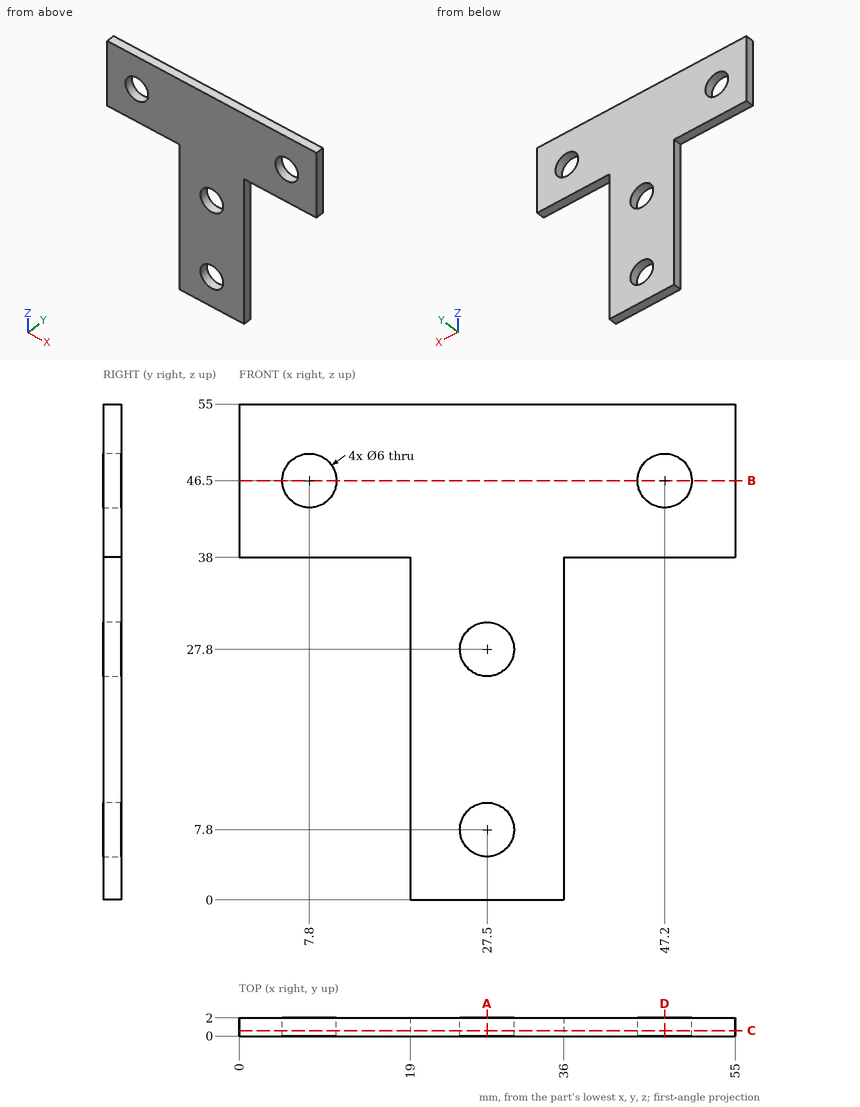
Source: three-view drawing plus pictorial views. Frame: mm from the lowest corner of the part. Round coordinates to 2 decimals unless told otherwise and drop trailing zeros. Loops run counter-clockwise (first coordinate to the right, second up) from the corner with the lowest first, then second, coordinate; pieces in that order, holes last.
Q1. Material intervals for L1, parallel to X at y = 0.5, z = 46.5; L2, parallel to X at y = 1.65, z = 7.8; L3, parallel to Z at x = 30, y = 0.85, sorted ascending.
Q2. Section C-C on y = 0.6. Return loops of the section in (x, z), plus the area to 3 significant figures.
Q3. Section B-B on z = 46.5. Return loops of the section in (x, y), plus the area to 3 significant figures.
Q4. Section D-D on x = 47.2. Return loops of the section in (y, z).
Q5. Pin query (flat end, axial travel): P1, Ø3.5, axis at x = 7.8, z = 46.5, coming from the +Y side; P2, Ø1, axis at y = 1, z = 28.5, coming from the -X side; P3, Ø0.6, axis at x = 43, y = 1.5, coming from the -Z side; P4, Ø1, axis at y = 1, z = 11, coming from the +X side. Return the tip coordinate at first contact, or that it passes through.
Q6. Section A-A on x = 27.5. Return loops of the section in (y, z).
Evaluation:
1. L1: x = 0 to 4.8, 10.8 to 44.2, 50.2 to 55
1. L2: x = 19 to 24.5, 30.5 to 36
1. L3: z = 0 to 6.14, 9.46 to 26.14, 29.46 to 55
2. outline: (0, 38) - (19, 38) - (19, 0) - (36, 0) - (36, 38) - (55, 38) - (55, 55) - (0, 55) - close; hole circle Ø6 at (7.8, 46.5); hole circle Ø6 at (27.5, 7.8); hole circle Ø6 at (27.5, 27.8); hole circle Ø6 at (47.2, 46.5)
2. area: 1,470 mm2
3. outline: (0, 0) - (4.8, 0) - (4.8, 2) - (0, 2) - close; (10.8, 0) - (44.2, 0) - (44.2, 2) - (10.8, 2) - close; (50.2, 0) - (55, 0) - (55, 2) - (50.2, 2) - close
3. area: 86.0 mm2
4. outline: (0, 38) - (2, 38) - (2, 43.5) - (0, 43.5) - close; (0, 49.5) - (2, 49.5) - (2, 55) - (0, 55) - close
5. P1: passes through
5. P2: stops at x = 19
5. P3: stops at z = 38
5. P4: stops at x = 36
6. outline: (0, 0) - (2, 0) - (2, 4.8) - (0, 4.8) - close; (0, 10.8) - (2, 10.8) - (2, 24.8) - (0, 24.8) - close; (0, 30.8) - (2, 30.8) - (2, 55) - (0, 55) - close
